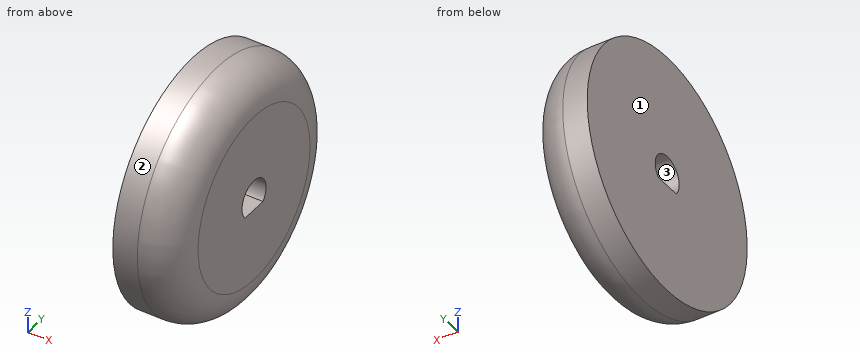
```python
from build123d import *

# Parameters (mm, degrees)
SKETCH1_R           = 10
BOSS_EXTRUDE1_DEPTH = 10
CUT_EXTRUDE1_DEPTH  = 18.320508076
FILLET1_R           = 3


with BuildPart() as part:
    # Sketch1 → Boss-Extrude1 (new body)
    with BuildSketch(Plane(origin=(0, 0, 0), x_dir=(0, -1, 0), z_dir=(1, 0, 0))):
        with Locations(Location((0, 0, 0), (0, 0, 90))):
            Circle(SKETCH1_R)
    extrude(amount=BOSS_EXTRUDE1_DEPTH)

    # Sketch2 → Cut-Extrude1 (cut, through all)
    with BuildSketch(Plane(origin=(10, 0, 0), x_dir=(0, -1, 0), z_dir=(1, 0, 0))):
        with BuildLine():
            Line((-1.118033989, 1), (1.118033989, 1))
            ThreePointArc((1.118033989, 1), (0, -1.5), (-1.118033989, 1))
        make_face()
    extrude(amount=-CUT_EXTRUDE1_DEPTH, mode=Mode.SUBTRACT)

    # Fillet1
    fillet1_edges = [part.edges().sort_by_distance(p)[0] for p in [
        (0, 0, 10),
        (10, 0, 10),
    ]]
    fillet(fillet1_edges, radius=FILLET1_R)

    # SurfaceCut1
    split(bisect_by=Plane.ZY.offset(-5), keep=Keep.BOTTOM)


solid = part.part
```
The listing builds one solid part. Answer for the finished solid, in the listing's coordinates (mm). Face numbers are marked on the shaded views. Round coordinates to 2 decimals unless told otherwise and drop trailing zeros. Write each loop counter-clockwise with the first axis right and the second up, starting at its lowest first coordinate (ties: lowest second). Pieces come first, ordered by that corner, then holes. Notation, with made-up numbers: (-14, 37) -> (18, 37) arc R22 ccw to (18, 45) -> close; hole circle Ø9 at (-24.5, 16). An arc over 180 degrees is marked (long way). Use CSV: the item, a comma, the result in double quotes. Start each with the question number.
(1) The mould has two halves that part along Y. Classify the marked faces 1, 2 and 3: released by +Y, released by -Y, zero draft, split by the parting line, or undercut.
(2) Section D-D on x = 8.15 is taken. Give the vertices of the cut face in (y, z), then the cut area to 3 significant figures.
(3) Section C-C on x = 5.65 is taken. Give the vertices of the cut face in (y, z).
(4) Section B-B on z = 0 is taken. Give the vertices of the cut face in (x, y), then the cut area to 3 significant figures.
(5) Consider L1, parallel to Y at x = 6.25, z = 0; L2, parallel to Y at x = 9.2, z = 0; L3, parallel to Z at x = 8.95, y = 8.5. Determine where each line is inside the solid, lowest interval first. Write a range as from..to.
(6) Section A-A on y = 0 is taken. Give the vertices of the cut face in (x, z).
(7) Each of these flat-tipped pins is pushed along its axis until it touches: pin 1 (3 mm diameter, centred on x = 6.5, y = -4.5, fed in from +Z); pin 2 (3.5 mm diameter, centred on y = 0, z = 0, fed in from +X); pin 3 (1.5 mm diameter, centred on x = 8, y = -5, fed in from -Z); pin 4 (0.7 mm diameter, centred on x = 8.5, y = 0.5, fed in from +Z). Where does it stop, or does it pass through?
A:
1,face 1,"zero draft"
1,face 2,"split by the parting line"
1,face 3,"undercut"
2,outline,"circle Ø19.54 at (0, 0); hole (-1.12, -1) -> (1.12, -1) arc R1.5 ccw (long way) to start"
2,area,"294 mm²"
3,outline,"circle Ø20 at (0, 0); hole (-1.12, -1) -> (1.12, -1) arc R1.5 ccw (long way) to start"
4,outline,"(5, -10) -> (7, -10) arc R3 ccw to (10, -7) -> (10, -1.5) -> (5, -1.5) -> close; (5, 1.5) -> (10, 1.5) -> (10, 7) arc R3 ccw to (7, 10) -> (5, 10) -> close"
4,area,"81.1 mm²"
5,L1,"y = -10..-1.5, 1.5..10"
5,L2,"y = -9.04..-1.5, 1.5..9.04"
5,L3,"z = -3.72..3.72"
6,outline,"(5, -10) -> (7, -10) arc R3 ccw to (10, -7) -> (10, -1) -> (5, -1) -> close; (5, 1.5) -> (10, 1.5) -> (10, 7) arc R3 ccw to (7, 10) -> (5, 10) -> close"
7,pin 1,"stops at z = 9.54"
7,pin 2,"stops at x = 10"
7,pin 3,"stops at z = -8.93"
7,pin 4,"stops at z = 9.76"
